```python
from build123d import *

# Parameters (mm, degrees)
BOSS_EXTRUDE1_DEPTH = 20


with BuildPart() as part:
    # Sketch1 → Boss-Extrude1 (new body, symmetric)
    with BuildSketch(Plane.XY):
        with BuildLine():
            Line((0, 4), (0, 25))
            Line((0, 25), (2, 25))
            Line((2, 25), (2, 4))
            ThreePointArc((2, 4), (2.585786438, 2.585786438), (4, 2))
            Line((4, 2), (25, 2))
            Line((25, 2), (25, 0))
            Line((25, 0), (4, 0))
            ThreePointArc((4, 0), (1.171572875, 1.171572875), (0, 4))
        make_face()
    extrude(amount=BOSS_EXTRUDE1_DEPTH, both=True)


solid = part.part
```
For this review, take the finished solid that the model builds, in its own axes (mm). A direction names the side the tool comes from. Give positions to 0.01 mm unless a question says otherwise; leave off trailing zeros. Order: outer loops, then holes, each group sorted by start corner. A loop starts at its lowest first (then second) coordinate and runs counter-clockwise, first axis right, second up.
1) Take a section at A-A (z = -12). Give the boundary of the cut face in (x, y), then the cut area to 3 significant figures.
2) Take a section at B-B (y = 9). Give the boundary of the cut face in (x, z).
3) Insertion check: pin 1 (6 mm diameter, centred on y = 13, z = -0.5, fed in from +X); pin 2 (1 mm diameter, centred on x = 8, z = -13, fed in from +Y). Each pin has a flat end and moves straight along its axis. Give the tip position at first contact, or say it passes through.
4) Wall thickness on line 1 (Y direction, x = 22.25, z = 8.5); line 2 (X direction, y = 2.25, z = 1.5): over which ranges is each line inside the solid? List them lowest first.
5) For faces 1 (the face through (7, 1, 20)), 2 (the face through (2, 15, 0)), list the 3-axis set-ups (+Z, -Z, +X, -X, +Y, -Y) from which the entire face can be reached by the end or side of a thin tool; tool diameter is ignored.
Derived:
1. outline: (0, 4) arc R4 ccw to (4, 0) - (25, 0) - (25, 2) - (4, 2) arc R2 cw to (2, 4) - (2, 25) - (0, 25) - close
1. area: 93.4 mm2
2. outline: (0, -20) - (2, -20) - (2, 20) - (0, 20) - close
3. pin 1: stops at x = 2
3. pin 2: stops at y = 2
4. line 1: y = 0 to 2
4. line 2: x = 0.4 to 3.03
5. face 1: +Z, +X, -X, +Y, -Y
5. face 2: +Z, -Z, +X, +Y
